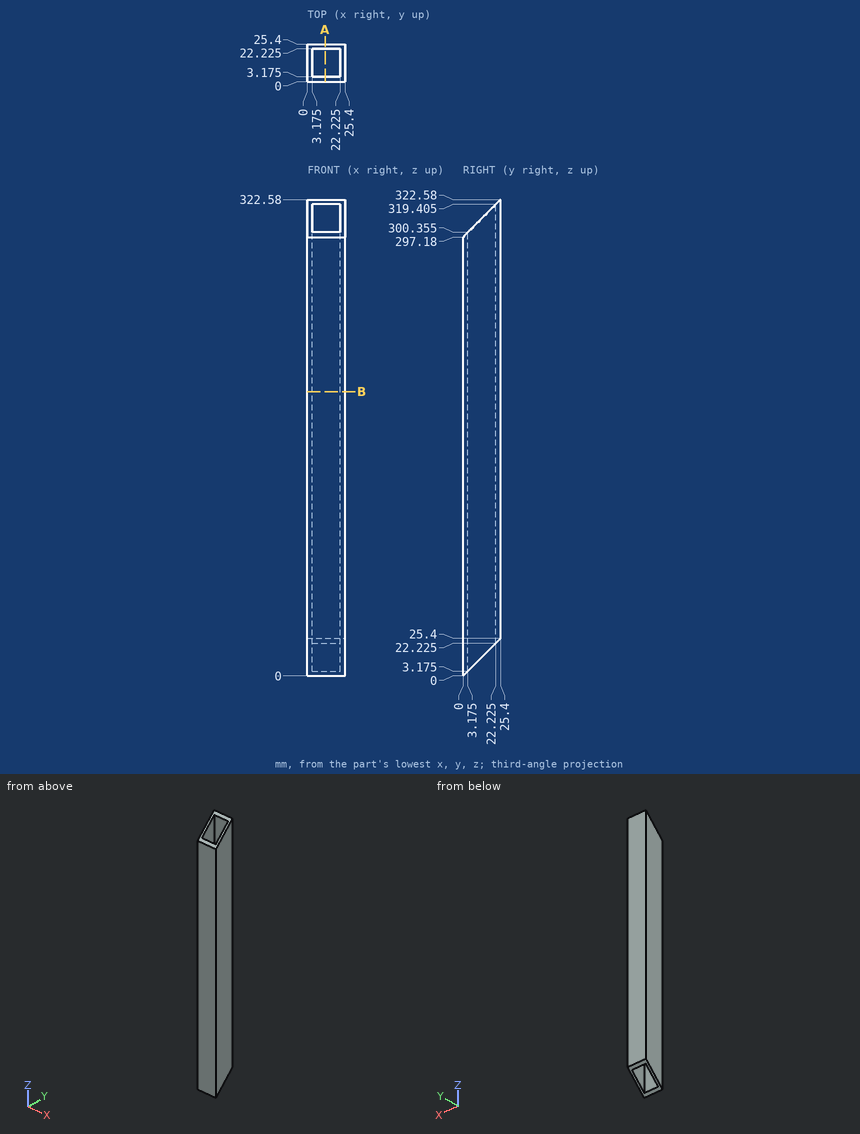
Geometry check sheet. Reference: drawing and pictorial views, mm from the part's lowest x, y, z. Round coordinates to 2 decimals unless told otherwise and drop trailing zeros. Write each loop counter-clockwise with the first axis right and the second up, starting at its lowest first coordinate (ties: lowest second). Pieces come first, ordered by that corner, then holes.
1. Section check B-B on z = 192.5. Enter the section's corners in (x, y) (3 decimals), plus the area to 3 significant figures.
2. Gauge pin test, flat ends, axial feed: P1, Ø8, axis at x = 14, y = 19.5, coming from the -Z side (3 decimals); P2, Ø6, axis at x = 19, y = 6.5, coming from the -Z side; P3, Ø4, axis at x = 3.5, y = 21, coming from the +Z side. Record the tip position at first contact, or that the pin passes through.
3. Scan lines: L1, parallel to Y at x = 21.75, z = 74.5 (3 decimals); L2, parallel to Y at x = 15.25, z = 309 (3 decimals). Record each from-to range of solid material in increasing order.
4. Section check A-A on x = 12. Enter the section's corners in (y, z) (3 decimals), plus the area to 3 significant figures.
Answer:
1. outline: (0, 0) - (25.4, 0) - (25.4, 25.4) - (0, 25.4) - close; hole (3.175, 3.175) - (22.225, 3.175) - (22.225, 22.225) - (3.175, 22.225) - close
1. area: 282 mm2
2. P1: stops at z = 22.225
2. P2: passes through
2. P3: stops at z = 320.18
3. L1: y = 0 to 3.175, 22.225 to 25.4
3. L2: y = 22.225 to 25.4
4. outline: (0, 0) - (3.175, 3.175) - (3.175, 300.355) - (0, 297.18) - close; (22.225, 22.225) - (25.4, 25.4) - (25.4, 322.58) - (22.225, 319.405) - close
4. area: 1,890 mm2
